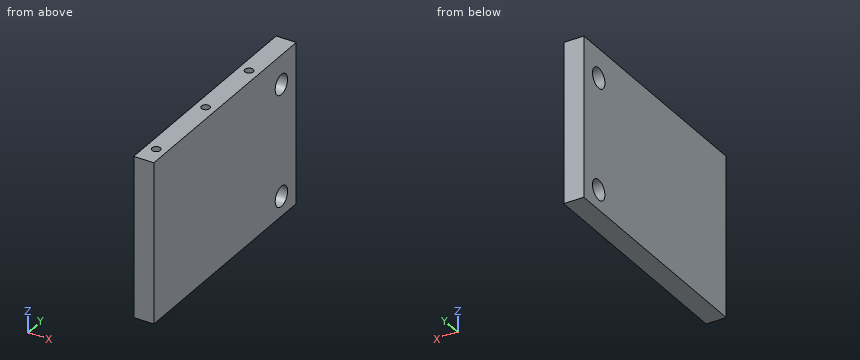
Autodesk Inventor part; units mm, degrees
ref_plane "YZ Plane" through (0, 0, 0) normal (1, 0, 0) x (0, 1, 0)
ref_plane "XZ Plane" through (0, 0, 0) normal (0, 1, 0) x (-1, 0, 0)
ref_plane "XY Plane" through (0, 0, 0) normal (0, 0, 1) x (1, 0, 0)
sketch "Skizze1" plane through (0, 0, 0) normal (0, 0, 1) x (1, 0, 0)
  line L0 (0, 0) -> (10, 0)
  line L1 (10, 0) -> (10, 115)
  line L2 (10, 115) -> (0, 115)
  line L3 (0, 115) -> (0, 0)
  dimension "d0" = 10
  dimension "d1" = 115
extrude "Extrusion1" add sketch "Skizze1" along normal blind 80
sketch "Skizze2" plane through (0, 0, 0) normal (-1, 0, 0) x (0, 0, 1)
  line L0 (0, 0) -> (0, 115)
  line L1 (0, 115) -> (0, 103)
  line L2 (0, 103) -> (9.875, 103)
  line L3 (9.875, 103) -> (65.375, 103)
  dimension "d4" = 12
  dimension "d5" = 9.875
  dimension "d6" = 55.5
hole "Bohrung1" at (0, 103, 9.875) at (0, 103, 65.375) direction (1, 0, 0) diameter 10 end through all
sketch "Skizze3" plane through (0, 0, 80) normal (0, 0, 1) x (1, 0, 0)
  line L0 (10, 115) -> (0, 115)
  line L1 (5, 115) -> (5, 85)
  line L2 (5, 85) -> (5, 50)
  line L3 (5, 50) -> (5, 10)
  point P0 (0, 0)
  dimension "d14" = 30
  dimension "d15" = 35
  dimension "d16" = 40
hole "Bohrung2" at (5, 85, 80) at (5, 10, 80) at (5, 50, 80) direction (0, 0, -1) diameter 4.134 depth 14.2 tip angle 118
properties part number "Motorhalterung_Grundplatte" material "Aluminium 6061"
CAD build for the part. Positions are in the model's coordinates, mm. Round coordinates to 2 decimals unless told otherwise and drop trailing zeros. Write each loop counter-clockwise with the first axis right and the second up, starting at its lowest first coordinate (ties: lowest second). Pieces come first, ordered by that corner, then holes. Notation, with made-up numbers: M 58.25,17 L 98.25,17 A7 cw 98.25,27 Z; hole C -31.5,-9 d1. An arc over 180 degrees is marked long. Use a Markdown table: item, result. Add a question column.
1. Slice it at A-A on y = 103. Give the cut face in (x, z) (3 decimals).
2. Drill centre lines: probe 1 along Z at (x, y) = (4.25, 103) (3 decimals); probe 2 along Y at (x, z) = (5, 77); probe 3 along X at (y, z) = (10, 74.75). Where is each one in solid material? Low to high.
3. Flat gauge pins, fed straight in: P1, Ø5, axis at x = 7.5, y = 16, coming from the -Z side; P2, Ø3.5, axis at x = 5, y = 85, coming from the +Z side. Where does each tip first touch, or does it go through?
Reply:
| question | item | result |
|---|---|---|
| 1 | outline | M 0,0 L 10,0 L 10,4.875 L 0,4.875 Z; M 0,14.875 L 10,14.875 L 10,60.375 L 0,60.375 Z; M 0,70.375 L 10,70.375 L 10,80 L 0,80 Z |
| 2 | probe 1 | z = 0 to 4.875, 14.875 to 60.375, 70.375 to 80 |
| 2 | probe 2 | y = 0 to 7.93, 12.07 to 47.93, 52.07 to 82.93, 87.07 to 115 |
| 2 | probe 3 | x = 0 to 2.93, 7.07 to 10 |
| 3 | P1 | stops at z = 0 |
| 3 | P2 | stops at z = 65.61 |
